Design review of the part built by this model. Coordinates are the model's own, in mm. Round coordinates to 2 decimals unless told otherwise and drop trailing zeros. Loops run counter-clockwise (first coordinate to the right, second up) from the corner with the lowest first, then second, coordinate; pieces in that order, holes last. Notation, with made-up numbers: (76.5, 36.5) - (127.5, 36.5) arc R10 ccw to (127.5, 54.5) - close; hole circle Ø1 at (30, -0.75). An arc over 180 degrees is marked (long way). Use one line per item in the form item = value. Start each with the question number.
(1) We need section D-D, the plane z = 9.3. Write out the cut boundary in (x, y), then the cut area to 3 significant figures.
(2) Wall thickness on probe 1 along Z at (x, y) = (-15.5, 1.9); probe 2 along Z at (x, y) = (-9.3, 2.05): over which ranges is each line inside the solid? List them lowest first. Write a range as [from, to].
(3) We need section B-B, the plane z = 0. Write out the cut boundary in (x, y).
(4) For pin 1 (6.5 mm diameter, centred on x = 15.5, z = 15.5, fed in from -Y), flat-tipped, find the tip position at first contact; note if it passes through.
(5) We need section A-A, the plane x = -9.3. Write out the cut boundary in (y, z), then the cut area to 3 significant figures.
(6) We need section C-C, the plane x = 0. Write out the cut boundary in (y, z).
from build123d import *

# Parameters (mm, degrees)
SKETCH_1_W               = 42
SKETCH_1_H               = 42
EXTRUDE_1_DEPTH          = 3
SKETCH_2_R               = 6
CUT_EXTRUDE_1_DEPTH      = 4
SKETCH_4_R               = 2.1
CUT_EXTRUDE_2_DEPTH      = 4
SKETCH_5_R               = 2.1
CUT_EXTRUDE_3_DEPTH      = 4
PATTERN_CIRCULAR_1_COUNT = 4
CHAMFER_1_SIZE           = 1


with BuildPart() as part:
    # 草圖1 → 填料-伸長1 (new body)
    with BuildSketch(Plane(origin=(0, 0, 0), x_dir=(1, 0, 0), z_dir=(0, 1, 0))):
        Rectangle(SKETCH_1_W, SKETCH_1_H)
    extrude(amount=EXTRUDE_1_DEPTH)

    # 草圖2 → 除料-伸長1 (cut, through all)
    with BuildSketch(Plane.XZ):
        Circle(SKETCH_2_R)
    extrude(amount=-CUT_EXTRUDE_1_DEPTH, mode=Mode.SUBTRACT)

    # 草圖4 → 除料-伸長2 (cut, through all)
    with BuildSketch(Plane(origin=(0, 3, 0), x_dir=(1, 0, 0), z_dir=(0, 1, 0))):
        with Locations((-9.3, 9.3)):
            Circle(SKETCH_4_R)
    cut_extrude_2 = extrude(amount=-CUT_EXTRUDE_2_DEPTH, mode=Mode.SUBTRACT)

    # 草圖5 → 除料-伸長3 (cut, through all)
    with BuildSketch(Plane(origin=(0, 3, 0), x_dir=(1, 0, 0), z_dir=(0, 1, 0))):
        with Locations((-15.5, 15.5)):
            Circle(SKETCH_5_R)
    cut_extrude_3 = extrude(amount=-CUT_EXTRUDE_3_DEPTH, mode=Mode.SUBTRACT)

    # 環狀複製排列1: 除料-伸長2, 除料-伸長3 ×4 about axis
    pattern_circular_1_axis = Axis((0, 0, 0), (0, 1, 0))
    for i in range(1, PATTERN_CIRCULAR_1_COUNT):
        add(cut_extrude_2.rotate(pattern_circular_1_axis, i * 360 / PATTERN_CIRCULAR_1_COUNT), mode=Mode.SUBTRACT)
        add(cut_extrude_3.rotate(pattern_circular_1_axis, i * 360 / PATTERN_CIRCULAR_1_COUNT), mode=Mode.SUBTRACT)

    # 導角1
    chamfer_1_edges = [part.edges().sort_by_distance(p)[0] for p in [
        (21, 1.5, 21),
        (-21, 1.5, 21),
        (-21, 1.5, -21),
        (21, 1.5, -21),
    ]]
    chamfer(chamfer_1_edges, length=CHAMFER_1_SIZE)


solid = part.part
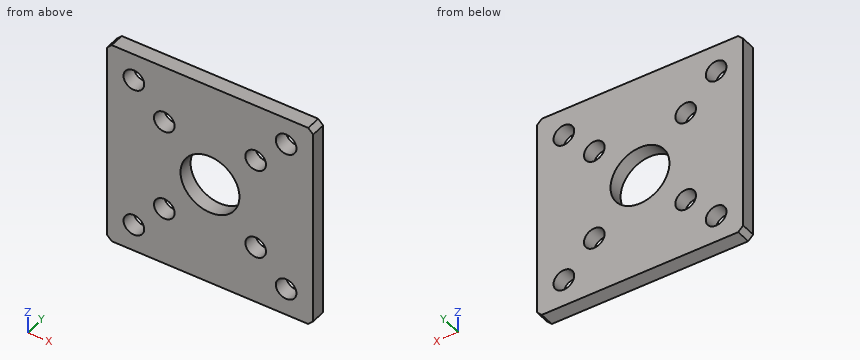
Data:
q1.outline = (-21, 0) - (-11.4, 0) - (-11.4, 3) - (-21, 3) - close; (-7.2, 0) - (7.2, 0) - (7.2, 3) - (-7.2, 3) - close; (11.4, 0) - (21, 0) - (21, 3) - (11.4, 3) - close
q1.area = 101 mm^2
q2.probe_1 = [-21, -17.6], [-13.4, 13.4], [17.6, 21]
q2.probe_2 = [-21, -11.4], [-7.2, 7.2], [11.4, 21]
q3.outline = (-21, 0) - (-6, 0) - (-6, 3) - (-21, 3) - close; (6, 0) - (21, 0) - (21, 3) - (6, 3) - close
q4.pin_1 = 0
q5.outline = (0, -21) - (3, -21) - (3, -11.4) - (0, -11.4) - close; (0, -7.2) - (3, -7.2) - (3, 7.2) - (0, 7.2) - close; (0, 11.4) - (3, 11.4) - (3, 21) - (0, 21) - close
q5.area = 101 mm^2
q6.outline = (0, -21) - (3, -21) - (3, -6) - (0, -6) - close; (0, 6) - (3, 6) - (3, 21) - (0, 21) - close
